Verification items for the finished model (mm, model axes). A direction names the side the tool comes from. Coordinates: 2 decimals unless noted, no trailing zeros. Write each loop counter-clockwise with the first axis right and the second up, starting at its lowest first coordinate (ties: lowest second). Pieces come first, ordered by that corner, then holes. Notation, with made-up numbers: (62.25, 86.5) -> (96.25, 86.5) arc R26 ccw to (96.25, 119.5) -> close; hole circle Ø5 at (45.5, 52.5). An arc over 180 degrees is marked (long way). Write item = value, one per line. Start each with the question number.
(1) Mould release check, pull along X, two halves, no side actions. Record for faces 1 (the face through (-3.04, 8.18, 473.48)), 2 (the face through (210.29, 5, 233)), 3 (the face through (212.307, 6.412, 473.479)), 4 (the face through (103, 5, 475)): released by +X, released by -X, zero draft, split by the parting line, or undercut.
(2) Material ranges on probe 1 along Y at (x, z) = (-6.5, 473.2); probe 2 along Y at (x, z) = (137.5, 237.5); probe 3 along X at (y, z) = (3.5, 397.5), recorded low to high. Write a range as [from, to].
(3) Gauge pin test, flat ends, axial feed: pin 1 Ø6 at (y, z) = (5.5, 53) entering from +X; pin 2 Ø7.5 at (x, y) = (-6.5, 5) entering from -Z; pin 3 Ø3 at (y, z) = (4, 280) entering from -X; pin 4 Ø5 at (x, z) = (44, 342) entering from -Y. Record the tip position at first contact, or that the pin passes through.
(4) Set-up check for faces 5 (the face through (222, 5, 472)), 6 (the face through (104, 5, 0)), 7 (the face through (-12, 5, 472)): record each of +Z, -Z, +X, -X, +Y, -Y from which the full face is reachable in a straight line by a thin tool's end or side.
(5) Section check B-B (x = 216.79). Record the cut outline in (y, z), plus the area to 3 significant figures.
(6) Section check D-D (x = 18). Record the cut outline in (y, z).
(7) Section check C-C (z = 392). Record the cut outline in (x, y).
(8) Section check A-A (y = 5). Record the cut outline in (x, z).
```python
from build123d import *

# Parameters (mm, degrees)
SKETCH1_W           = 210.29
SKETCH1_H           = 10
BOSS_EXTRUDE1_DEPTH = 475
SKETCH2_W           = 3
SKETCH2_H           = 15
BOSS_EXTRUDE2_DEPTH = 14
SKETCH4_W           = 3
SKETCH4_H           = 15
BOSS_EXTRUDE3_DEPTH = 14
SKETCH3_R           = 4.7
CUT_EXTRUDE1_DEPTH  = 13


with BuildPart() as part:
    # Sketch1 → Boss-Extrude1 (new body)
    with BuildSketch(Plane.XY):
        with Locations((105.145, 5)):
            Rectangle(SKETCH1_W, SKETCH1_H)
    extrude(amount=BOSS_EXTRUDE1_DEPTH)

    # Sketch2 → Boss-Extrude2 (add)
    with BuildSketch(Plane.ZY):
        with Locations((473.5, 5)):
            Rectangle(SKETCH2_W, SKETCH2_H)
    extrude(amount=BOSS_EXTRUDE2_DEPTH)

    # Sketch4 → Boss-Extrude3 (add)
    with BuildSketch(Plane(origin=(210.29, 0, 0), x_dir=(0, 0, -1), z_dir=(1, 0, 0))):
        with Locations((-473.5, 5)):
            Rectangle(SKETCH4_W, SKETCH4_H)
    extrude(amount=BOSS_EXTRUDE3_DEPTH)

    # Sketch3 → Cut-Extrude1 (cut)
    with BuildSketch(Plane(origin=(0, 0, 472), x_dir=(-1, 0, 0), z_dir=(0, 0, -1))):
        with Locations((6.5, 5)):
            Circle(SKETCH3_R)
        with Locations((-216.79, 5)):
            Circle(SKETCH3_R)
    extrude(amount=-CUT_EXTRUDE1_DEPTH, mode=Mode.SUBTRACT)


solid = part.part
```
Response:
q1.face_1 = undercut
q1.face_2 = released by +X
q1.face_3 = undercut
q1.face_4 = zero draft
q2.probe_1 = [-2.5, 0.3], [9.7, 12.5]
q2.probe_2 = [0, 10]
q2.probe_3 = [0, 210.29]
q3.pin_1 = 210.29
q3.pin_2 = through
q3.pin_3 = 0
q3.pin_4 = 0
q4.face_5 = -Z, +X, +Y, -Y
q4.face_6 = -Z, +X, -X, +Y, -Y
q4.face_7 = -Z, -X, +Y, -Y
q5.outline = (-2.5, 472) -> (0.3, 472) -> (0.3, 475) -> (-2.5, 475) -> close; (9.7, 472) -> (12.5, 472) -> (12.5, 475) -> (9.7, 475) -> close
q5.area = 16.8 mm2
q6.outline = (0, 0) -> (10, 0) -> (10, 475) -> (0, 475) -> close
q7.outline = (0, 0) -> (210.29, 0) -> (210.29, 10) -> (0, 10) -> close
q8.outline = (-14, 472) -> (-11.2, 472) -> (-11.2, 475) -> (-14, 475) -> close; (-1.8, 472) -> (0, 472) -> (0, 0) -> (210.29, 0) -> (210.29, 472) -> (212.09, 472) -> (212.09, 475) -> (-1.8, 475) -> close; (221.49, 472) -> (224.29, 472) -> (224.29, 475) -> (221.49, 475) -> close
